Here's how the part is built. I have some questions about the finished solid (model axes, mm). Coordinates: 2 decimals unless noted, no trailing zeros. Loops run counter-clockwise (first coordinate to the right, second up) from the corner with the lowest first, then second, coordinate; pieces in that order, holes last. Notation, with made-up numbers: (-35, 20) - (0, 20) arc R9 cw to (0, 25) - close; hole circle Ø1 at (84.25, 49). An arc over 180 degrees is marked (long way). Use a Markdown table: item, result.
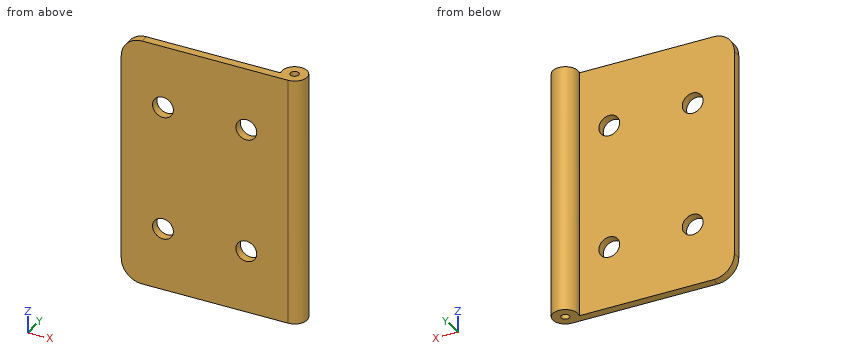
```python
from build123d import *

# Parameters (mm, degrees)
SKETCH1_W           = 40
SKETCH1_H           = 60
SKETCH1_R           = 2.5
BOSS_EXTRUDE1_DEPTH = 2
FILLET1_R           = 5
SKETCH2_R           = 3
SKETCH2_R_2         = 1
BOSS_EXTRUDE2_DEPTH = 60


with BuildPart() as part:
    # Sketch1 → Boss-Extrude1 (new body)
    with BuildSketch(Plane(origin=(0, 0, 0), x_dir=(1, 0, 0), z_dir=(0, 1, 0))):
        with Locations((-20, 0)):
            Rectangle(SKETCH1_W, SKETCH1_H)
        with Locations((-30, 15)):
            Circle(SKETCH1_R, mode=Mode.SUBTRACT)
        with Locations((-10, 15)):
            Circle(SKETCH1_R, mode=Mode.SUBTRACT)
        with Locations((-10, -15)):
            Circle(SKETCH1_R, mode=Mode.SUBTRACT)
        with Locations((-30, -15)):
            Circle(SKETCH1_R, mode=Mode.SUBTRACT)
    extrude(amount=BOSS_EXTRUDE1_DEPTH)

    # Fillet1
    fillet1_edges = [part.edges().sort_by_distance(p)[0] for p in [
        (-40, 1, 30),
        (-40, 1, -30),
    ]]
    fillet(fillet1_edges, radius=FILLET1_R)

    # Sketch2 → Boss-Extrude2 (add)
    with BuildSketch(Plane.XY.offset(30)):
        with Locations((0, 3)):
            Circle(SKETCH2_R)
        with Locations((0, 3)):
            Circle(SKETCH2_R_2, mode=Mode.SUBTRACT)
    extrude(amount=-BOSS_EXTRUDE2_DEPTH)


solid = part.part
```
Q1. Will these pins go through, and if not, where does the flat tip stop? P1, Ø3, axis at y = 1.5, z = 11.5, coming from the +X side; P2, Ø6.5, axis at x = -30, z = 15, coming from the +Y side; P3, Ø1, axis at y = 1, z = 21, coming from the +X side.
Check values:
| item | result |
|---|---|
| P1 | x = 3 |
| P2 | y = 2 |
| P3 | x = 2.6 |
Q2. I want a section at B-B, the plane x = -30. Write out the boundary of the cut face in (y, z), then the cut area to 3 significant figures.
Check values:
| item | result |
|---|---|
| outline | (0, -30) - (2, -30) - (2, -17.5) - (0, -17.5) - close; (0, -12.5) - (2, -12.5) - (2, 12.5) - (0, 12.5) - close; (0, 17.5) - (2, 17.5) - (2, 30) - (0, 30) - close |
| area | 100 mm^2 |
Q3. I want a section at C-C, the plane y = 0.8. Write out the boundary of the cut face in (x, z), then the cut area to 3 significant figures.
Check values:
| item | result |
|---|---|
| outline | (-40, -25) arc R5 ccw to (-35, -30) - (2.04, -30) - (2.04, 30) - (-35, 30) arc R5 ccw to (-40, 25) - close; hole circle Ø5 at (-30, -15); hole circle Ø5 at (-30, 15); hole circle Ø5 at (-10, -15); hole circle Ø5 at (-10, 15) |
| area | 2,430 mm^2 |
Q4. Please list where these lines run through material, in increasing order: L1, parallel to Z at x = -10, y = 1.1; L2, parallel to Y at x = -34, z = -3; L3, parallel to X at y = 0.75, z = -15. Write a range as from..to.
Check values:
| item | result |
|---|---|
| L1 | -30..-17.5, -12.5..12.5, 17.5..30 |
| L2 | 0..2 |
| L3 | -40..-32.5, -27.5..-12.5, -7.5..1.98 |
Q5. I want a section at D-D, the plane z = -18.5. Write out the boundary of the cut face in (x, y), then the cut area to 3 significant figures.
Check values:
| item | result |
|---|---|
| outline | (-40, 0) - (0, 0) arc R3 ccw (long way) to (-2.83, 2) - (-40, 2) - close; hole circle Ø2 at (0, 3) |
| area | 101 mm^2 |
Q6. I want a section at A-A, the plane z = 15. Write out the boundary of the cut face in (x, y).
Check values:
| item | result |
|---|---|
| outline | (-40, 0) - (-32.5, 0) - (-32.5, 2) - (-40, 2) - close; (-27.5, 0) - (-12.5, 0) - (-12.5, 2) - (-27.5, 2) - close; (-7.5, 0) - (0, 0) arc R3 ccw (long way) to (-2.83, 2) - (-7.5, 2) - close; hole circle Ø2 at (0, 3) |
